```python
from build123d import *

# Parameters (mm, degrees)
POCKET001_DEPTH       = 111.6
POLARPATTERN001_COUNT = 4
SKETCH018_W           = 12.6
SKETCH018_H           = 33
POCKET002_DEPTH       = 111.6
POLARPATTERN002_COUNT = 4
SKETCH019_W           = 12.6
SKETCH019_H           = 24.2
POCKET003_DEPTH       = 920.1486
POLARPATTERN003_COUNT = 4
SKETCH020_R           = 0.75
POCKET004_DEPTH       = 121.6
POLARPATTERN004_COUNT = 4
SKETCH021_W           = 10
SKETCH021_H           = 30
POCKET005_DEPTH       = 920.1486
POLARPATTERN005_COUNT = 4


with BuildPart() as part:
    # Sketch → Revolution (revolve)
    with BuildSketch(Plane.XZ):
        with BuildLine():
            Line((110.527128, -120.57), (130.678, -120.57))
            Line((130.678, -120.57), (130.678, -2))
            ThreePointArc((130.678, -2), (110.678, 18), (90.678, -2))
            Line((90.678, -2), (90.678, -8))
            Line((90.678, -8), (110.527128, -120.57))
        make_face()
    revolve(axis=Axis((0, 0, 0), (0, 0, 1)))

    # Sketch017 → Pocket001 (cut)
    with BuildSketch(Plane.YZ):
        with BuildLine():
            ThreePointArc((-4.1, -148.6), (0, -152.7), (4.1, -148.6))
            Line((4.1, -148.6), (4.1, -28.6))
            ThreePointArc((4.1, -28.6), (0, -24.5), (-4.1, -28.6))
            Line((-4.1, -148.6), (-4.1, -28.6))
        make_face()
    pocket001 = extrude(amount=-POCKET001_DEPTH, mode=Mode.SUBTRACT)

    # PolarPattern001: Pocket001 ×4 about axis
    polarpattern001_axis = Axis((0, 0, 0), (0, 0, 1))
    for i in range(1, POLARPATTERN001_COUNT):
        add(pocket001.rotate(polarpattern001_axis, i * 360 / POLARPATTERN001_COUNT), mode=Mode.SUBTRACT)

    # Sketch018 → Pocket002 (cut)
    with BuildSketch(Plane.YZ):
        with Locations((0, -87)):
            Rectangle(SKETCH018_W, SKETCH018_H)
    pocket002 = extrude(amount=-POCKET002_DEPTH, mode=Mode.SUBTRACT)

    # PolarPattern002: Pocket002 ×4 about axis
    polarpattern002_axis = Axis((0, 0, 0), (0, 0, 1))
    for i in range(1, POLARPATTERN002_COUNT):
        add(pocket002.rotate(polarpattern002_axis, i * 360 / POLARPATTERN002_COUNT), mode=Mode.SUBTRACT)

    # Sketch019 → Pocket003 (cut, through all)
    with BuildSketch(Plane.YZ):
        with Locations((0, -87)):
            Rectangle(SKETCH019_W, SKETCH019_H)
    pocket003 = extrude(amount=-POCKET003_DEPTH, mode=Mode.SUBTRACT)

    # PolarPattern003: Pocket003 ×4 about axis
    polarpattern003_axis = Axis((0, 0, 0), (0, 0, 1))
    for i in range(1, POLARPATTERN003_COUNT):
        add(pocket003.rotate(polarpattern003_axis, i * 360 / POLARPATTERN003_COUNT), mode=Mode.SUBTRACT)

    # Sketch020 → Pocket004 (cut)
    with BuildSketch(Plane.YZ):
        with Locations((0, -73.25)):
            Circle(SKETCH020_R)
        with Locations((0, -100.75)):
            Circle(SKETCH020_R)
    pocket004 = extrude(amount=-POCKET004_DEPTH, mode=Mode.SUBTRACT)

    # PolarPattern004: Pocket004 ×4 about axis
    polarpattern004_axis = Axis((0, 0, 0), (0, 0, 1))
    for i in range(1, POLARPATTERN004_COUNT):
        add(pocket004.rotate(polarpattern004_axis, i * 360 / POLARPATTERN004_COUNT), mode=Mode.SUBTRACT)

    # Sketch021 → Pocket005 (cut, through all)
    with BuildSketch(Plane.YZ):
        with Locations((0, 13)):
            Rectangle(SKETCH021_W, SKETCH021_H)
    pocket005 = extrude(amount=-POCKET005_DEPTH, mode=Mode.SUBTRACT)

    # PolarPattern005: Pocket005 ×4 about axis
    polarpattern005_axis = Axis((0, 0, 0), (0, 0, 1))
    for i in range(1, POLARPATTERN005_COUNT):
        add(pocket005.rotate(polarpattern005_axis, i * 360 / POLARPATTERN005_COUNT), mode=Mode.SUBTRACT)


solid = part.part
```
Here's how the part is built. I have some questions about the finished solid (model axes, mm). A direction names the side the tool comes from. Round coordinates to 2 decimals unless told otherwise and drop trailing zeros. Write each loop counter-clockwise with the first axis right and the second up, starting at its lowest first coordinate (ties: lowest second). Pieces come first, ordered by that corner, then holes.
Q1. If we section it at A-A on z = -82.5: Write out the boundary of the cut face in (x, y).
Q2. Please list where these lines run through material, in increasing order: probe 1 along Z at (x, y) = (0, 117); probe 2 along Y at (x, z) = (0, -5.25); probe 3 along X at (y, z) = (32.5, -104).
Q3. Which directions (+Z, -Z, +X, -X, +Y, -Y) give clear straight access to the entire face, cutting with the end or side of a thin tool? Please do faces 1 (the flat face through (0, -121, -99.1)), 2 (the flat face through (0, 111.6, -110)), 3 (the flat face through (121, 0, -74.9)), 4 (the flat face through (4.1, 105, -50)), 5 (the flat face through (-110, 5, 6)).
Q4. If we section it at B-B on z = -39.5: Write out the boundary of the cut face in (x, y), plus the area to 4 significant figures.
Q5. Will these pins go through, and if not, where does the flat tip stop? P1, Ø16, axis at x = -114, z = 9, coming from the +Y side; P2, Ø11, axis at x = -2.5, y = 119, coming from the +Z side; P3, Ø1, axis at y = -31.5, z = 4, coming from the -X side (3 decimals); P4, Ø8, axis at x = 76, y = -35.5, coming from the +Z side.
Q6. If we mould it in two halves opening along Y, with no side actions, what happens to faces 6 (the flat face through (-5, -110, 6)), 7 (the flat face through (-116, -6.3, -87))? For each: +Y half, -Y half, draft (parallel to the pull), parting line (faces both ways), or undercut.
Answer below:
1. outline: (-130.53, -6.3) arc R130.68 ccw to (-6.3, -130.53) - (-6.3, -103.62) arc R103.81 cw to (-103.62, -6.3) - close; (-130.53, 6.3) - (-103.62, 6.3) arc R103.81 cw to (-6.3, 103.62) - (-6.3, 130.53) arc R130.68 ccw to start; (6.3, -130.53) arc R130.68 ccw to (130.53, -6.3) - (103.62, -6.3) arc R103.81 cw to (6.3, -103.62) - close; (6.3, 103.62) arc R103.81 cw to (103.62, 6.3) - (130.53, 6.3) arc R130.68 ccw to (6.3, 130.53) - close
2. probe 1: z = -120.57 to -101.5, -100 to -99.1, -74.9 to -74, -72.5 to -2
2. probe 2: y = -130.68 to -90.68, 90.68 to 130.68
2. probe 3: x = -126.57 to -102.58, 102.58 to 126.57
3. face 1: +Y, -Y
3. face 2: none
3. face 3: +X, -X
3. face 4: -Z
3. face 5: +Z, +X, -X
4. outline: circle Ø261.36 at (0, 0); hole (-111.6, -4.1) - (-96.14, -4.1) arc R96.23 ccw to (-4.1, -96.14) - (-4.1, -111.6) - (4.1, -111.6) - (4.1, -96.14) arc R96.23 ccw to (96.14, -4.1) - (111.6, -4.1) - (111.6, 4.1) - (96.14, 4.1) arc R96.23 ccw to (4.1, 96.14) - (4.1, 111.6) - (-4.1, 111.6) - (-4.1, 96.14) arc R96.23 ccw to (-96.14, 4.1) - (-111.6, 4.1) - close
4. area: 24,050 mm2
5. P1: stops at y = 72.73
5. P2: stops at z = 17.69
5. P3: stops at x = -126.075
5. P4: passes through
6. face 6: draft
6. face 7: undercut
